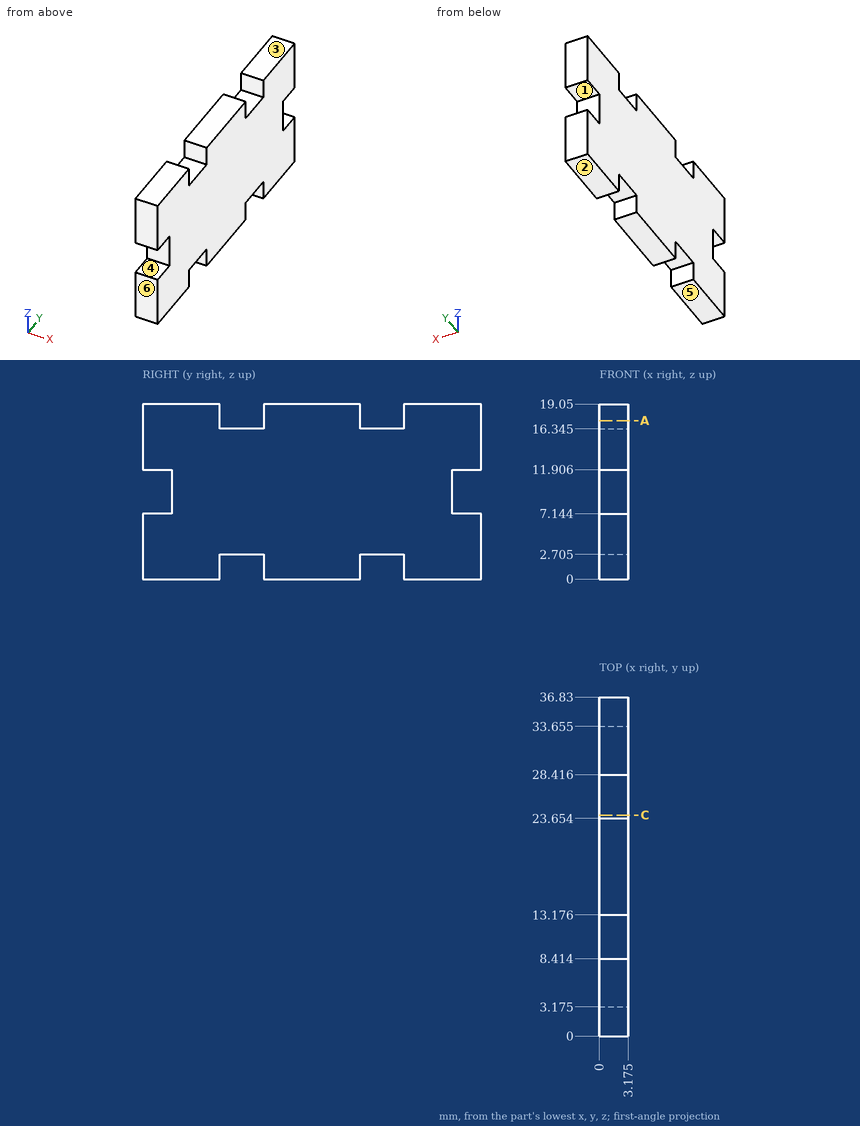
Geometry check sheet. Reference: drawing and pictorial views, mm from the part's lowest x, y, z. A direction names the side the tool comes from. Coordinates: 2 decimals unless noted, no trailing zeros. Order: outer loops, then holes, each group sorted by start corner. A loop starts at its lowest first (then second) coordinate and runs counter-clockwise, first axis right, second up.
1. Sectioned sample at A-A, the plane z = 17.25. Record the cut outline in (x, y) (1 decimal).
Results found:
outline: (0, 0) - (3.2, 0) - (3.2, 8.4) - (0, 8.4) - close; (0, 13.2) - (3.2, 13.2) - (3.2, 23.7) - (0, 23.7) - close; (0, 28.4) - (3.2, 28.4) - (3.2, 36.8) - (0, 36.8) - close
2. Go/stop test with flat-tipped pins: pin 1 Ø4 at (y, z) = (8, 13.5) entering from -X; pin 2 Ø1 at (x, y) = (1.5, 10.5) entering from +Z (1 decimal). Record where each tip stops, or that it passes through.
Results found:
pin 1: stops at x = 0
pin 2: stops at z = 16.3
3. Release check for a two-part mould opening along Z. For the marked faces 3, 4, 5 and 6 record: +Z half, -Z half, draft (parallel to the pull), parting line (faces both ways), or undercut.
Results found:
face 3: +Z half
face 4: undercut
face 5: -Z half
face 6: draft
4. Scan lines: line 1 (Y direction, x = 0.25, z = 17.25); line 2 (Z direction, x = 2.9, y = 27) (1 decimal); line 3 (Y direction, x = 0.95, z = 11.75) (1 decimal). Record each from-to range of solid material in increasing order.
Results found:
line 1: y = 0 to 8.41, 13.18 to 23.65, 28.42 to 36.83
line 2: z = 2.7 to 16.3
line 3: y = 3.2 to 33.7
5. Set-up check for the marked faces 1 and 2: record each of +Z, -Z, +X, -X, +Y, -Y from which the full face is reachable in a straight line by a thin tool's end or side.
Results found:
face 1: +X, -X, +Y
face 2: -Z, +X, -X, +Y, -Y
6. Sectioned sample at C-C, the plane y = 24. Record the cut outline in (x, z) (1 decimal), and give its area (3 significant figures).
Results found:
outline: (0, 2.7) - (3.2, 2.7) - (3.2, 16.3) - (0, 16.3) - close
area: 43.3 mm2
